Geometry: final body of the model. Coordinates: model frame, mm. A direction names the side the tool comes from. Give positions to 0.01 mm unless a question says otherwise; leave off trailing zeros. Write each loop counter-clockwise with the first axis right and the second up, starting at its lowest first coordinate (ties: lowest second). Pieces come first, ordered by that corner, then holes.
Q1. Section C-C (x = 87.5). Return the cut outline in (y, z), plus the area to 3 significant figures.
Q2. Line query: line 1 (X direction, y = 3.2, z = 7); line 2 (X direction, y = 12.75, z = 10); line 3 (Y direction, x = 87, z = 12.25). Output: solid intervals per line, ascending.
Q3. Mould query, pull axis X, two halves, no side actions, for faces 3 (the flat face through (57.503, 10, 9)), 4 (the cylindrical face through (127.575, 2.718, 6.35)), 5 (the flat face through (102, 4, 0)). Classes: +X half, -X half, draft (parallel to the pull), parting line (faces both ways), or undercut.
Q4. Section B-B (z = 7). Return the cut outline in (x, y), plus the area to 3 significant figures.
Q5. Reachability of faces 1 (the flat face through (142.503, 12, 9)), 2 (the flat face through (102, 4, 18)) from +Z, -Z, +X, -X, +Y, -Y: full face, straight path, thin tool, end or side. Return the list, or none.
Q6. Section A-A (y = 13.75). Return the cut outline in (x, z).
Q7. Pin query (flat end, axial travel): pin 1 Ø5.5 at (x, z) = (74.5, 7) entering from +Y; pin 2 Ø1.5 at (x, z) = (104.5, 14) entering from +Y. Return the tip coordinate at first contact, or that it passes through.
from build123d import *

# Parameters (mm, degrees)
SKETCH1_W           = 80
SKETCH1_H           = 18
SKETCH1_R           = 3
BOSS_EXTRUDE1_DEPTH = 5
SKETCH1_6_W         = 5
SKETCH1_6_H         = 18
BOSS_EXTRUDE2_DEPTH = 20
FILLET1_R           = 0.5


with BuildPart() as part:
    # Sketch1 → Boss-Extrude1 (new body)
    with BuildSketch(Plane(origin=(0, 0, 0), x_dir=(1, 0, 0), z_dir=(0, 1, 0))):
        with Locations((102.5033, -9)):
            Rectangle(SKETCH1_W, SKETCH1_H)
        with Locations(Location((74.5033, -7, 0), (0, 0, 270))):
            Circle(SKETCH1_R, mode=Mode.SUBTRACT)
        with Locations(Location((130.5033, -7, 0), (0, 0, 270))):
            Circle(SKETCH1_R, mode=Mode.SUBTRACT)
    extrude(amount=BOSS_EXTRUDE1_DEPTH)

    # Sketch1_6 → Boss-Extrude2 (add)
    with BuildSketch(Plane(origin=(0, 0, 0), x_dir=(1, 0, 0), z_dir=(0, 1, 0))):
        with Locations((60.0033, -9)):
            Rectangle(SKETCH1_6_W, SKETCH1_6_H)
        with Locations((145.0033, -9)):
            Rectangle(SKETCH1_6_W, SKETCH1_6_H)
    extrude(amount=BOSS_EXTRUDE2_DEPTH)

    # Fillet1
    fillet1_edges = [part.edges().sort_by_distance(p)[0] for p in [
        (74.5033, 0, 4),
        (130.5033, 0, 4),
        (57.5033, 0, 9),
        (57.5033, 10, 0),
        (57.5033, 10, 18),
        (57.5033, 20, 9),
        (147.5033, 20, 9),
        (147.5033, 10, 18),
        (147.5033, 10, 0),
        (147.5033, 0, 9),
        (102.5033, 0, 18),
        (102.5033, 0, 0),
    ]]
    fillet(fillet1_edges, radius=FILLET1_R)


solid = part.part
Computed:
1. outline: (0, 0.5) arc R0.5 ccw to (0.5, 0) - (5, 0) - (5, 18) - (0.5, 18) arc R0.5 ccw to (0, 17.5) - close
1. area: 89.9 mm2
2. line 1: x = 57.5 to 71.5, 77.5 to 127.5, 133.5 to 147.5
2. line 2: x = 57.5 to 62.5, 142.5 to 147.5
2. line 3: y = 0 to 5
3. face 3: -X half
3. face 4: undercut
3. face 5: draft
4. outline: (57.5, 0.5) arc R0.5 ccw to (58, 0) - (71, 0) arc R0.5 ccw to (71.5, 0.5) - (71.5, 5) - (62.5, 5) - (62.5, 20) - (58, 20) arc R0.5 ccw to (57.5, 19.5) - close; (77.5, 0.5) arc R0.5 ccw to (78, 0) - (127, 0) arc R0.5 ccw to (127.5, 0.5) - (127.5, 5) - (77.5, 5) - close; (133.5, 0.5) arc R0.5 ccw to (134, 0) - (147, 0) arc R0.5 ccw to (147.5, 0.5) - (147.5, 19.5) arc R0.5 ccw to (147, 20) - (142.5, 20) - (142.5, 5) - (133.5, 5) - close
4. area: 540 mm2
5. face 1: +Z, -Z, +Y
5. face 2: +Z, +X, -X, +Y, -Y
6. outline: (57.5, 0.5) arc R0.5 ccw to (58, 0) - (62.5, 0) - (62.5, 18) - (58, 18) arc R0.5 ccw to (57.5, 17.5) - close; (142.5, 0) - (147, 0) arc R0.5 ccw to (147.5, 0.5) - (147.5, 17.5) arc R0.5 ccw to (147, 18) - (142.5, 18) - close
7. pin 1: passes through
7. pin 2: stops at y = 5
